Can you work these out from the model? Positions are in its coordinate system, mm. Face numbers are marked on the shaded views. Round coordinates to 2 decimals unless told otherwise and drop trailing zeros. Loops run counter-clockwise (first coordinate to the right, second up) from the corner with the lowest first, then second, coordinate; pieces in that order, holes last. Notation, with made-up numbers: (-5.75, 77.25) -> (51.25, 77.25) arc R5 cw to (51.25, 86.25) -> close; hole circle Ø8 at (59.5, -16). An arc over 180 degrees is marked (long way). Write item = value, one per line.
Autodesk Inventor part; units mm, degrees
ref_plane "YZ Plane" through (0, 0, 0) normal (1, 0, 0) x (0, 1, 0)
ref_plane "XZ Plane" through (0, 0, 0) normal (0, 1, 0) x (-1, 0, 0)
ref_plane "XY Plane" through (0, 0, 0) normal (0, 0, 1) x (1, 0, 0)
sketch "Sketch1" plane through (0, 0, 0) normal (0, 0, 1) x (1, 0, 0)
  line L0 (0, 13.335) -> (0, -13.335)
  line L1 (-13.335, 0) -> (13.335, 0)
  circle A0 centre (0, 0) radius 9.525
  dimension "d0" = 19.05
extrude "Extrusion1" add sketch "Sketch1" along normal blind 6.35
sketch "Sketch2" plane through (0, 0, 6.35) normal (0, 0, 1) x (1, 0, 0)
  circle A0 centre (0, 0) radius 9.525
  circle A1 centre (0, 0) radius 4.7625
  dimension "d3" = 9.525
extrude "Extrusion2" cut sketch "Sketch2" against normal blind 2.54 contours A1
hole "Hole1" at (0, 0, 3.81) direction (0, 0, -1) diameter 4.4958 end through all countersink diameter 9.525 countersink angle 82
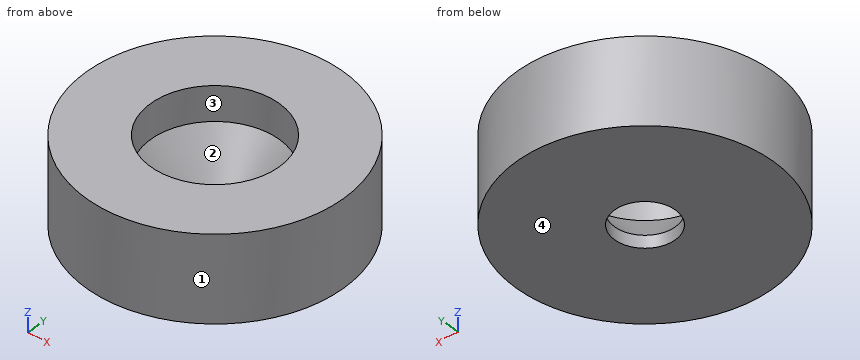
1. We'd pull the mould along X, two halves only. Please class the marked faces 1, 2, 3 and 4: released by +X, released by -X, zero draft, split by the parting line, or undercut.
Entries:
face_1 = split by the parting line
face_2 = undercut
face_3 = undercut
face_4 = zero draft
2. I need wall thicknesses on line 1 (Y direction, x = 0, z = 5.3) (1 decimal); line 2 (X direction, y = 0, z = 0.6) (3 decimals). Which ranges of each line are inside material? Lowest first, please. Write a range as [from, to].
Entries:
line_1 = [-9.5, -4.8], [4.8, 9.5]
line_2 = [-9.525, -2.248], [2.248, 9.525]
3. I'm going to push flat-ended pins straight in: pin 1 (4 mm diameter, centred on x = -3.5, y = 0, fed in from -Z); pin 2 (2 mm diameter, centred on y = 3.5, z = 5.5, fed in from +X); pin 3 (1 mm diameter, centred on x = -6, z = 2.5, fed in from +Y). Where does each tip first touch, or does it pass through?
Entries:
pin_1 = 0
pin_2 = 9.19
pin_3 = 7.78
4. Suppose I cut it at D-D, the plane x = -7.5. List the corners of the cut face in (y, z) for me.
Entries:
outline = (-5.87, 0) -> (5.87, 0) -> (5.87, 6.35) -> (-5.87, 6.35) -> close
